Read the model definition and answer for the solid it produces. Units are mm, in the model's axes. A direction names the side the tool comes from. Give positions to 0.01 mm unless a question says otherwise; leave off trailing zeros. Order: outer loops, then holes, each group sorted by start corner. A loop starts at its lowest first (then second) coordinate and runs counter-clockwise, first axis right, second up. Notation, with made-up numbers: M -40,83 L -24,83 A25 cw -24,117 Z; hole C -10,86 d7. An arc over 180 degrees is marked long. Write item = value, one per line. Start each with the question number.
from build123d import *

# Parameters (mm, degrees)
F0_R          = 55
F1_DEPTH      = 250
F1_DEPTH_BACK = 250
F3_DEPTH      = 12
F4_R          = 8
F5_R          = 2


with BuildPart() as f1:
    # F0 (on Right) → F1 (new body, two sides)
    with BuildSketch(Plane.YZ) as f1_sk:
        with Locations((-60, 100)):
            Circle(F0_R)
    extrude(amount=F1_DEPTH)
    extrude(f1_sk.sketch, amount=-F1_DEPTH_BACK)

    # F2 (on Right) → F3 (join)
    with BuildSketch(Plane.YZ):
        with BuildLine():
            ThreePointArc((-29.205577, 167.747019), (-18.607638, 166.4936), (-12.913269, 175.519204))
            Line((-12.913269, 175.519204), (-12.913269, 200))
            Line((-12.913269, 200), (-162.913269, 200))
            Line((-162.913269, 200), (-162.913269, 165))
            Line((-162.913269, 165), (-154.913269, 165))
            Line((-154.913269, 165), (-154.913269, 175))
            Line((-154.913269, 175), (-138.813269, 175))
            Line((-138.813269, 175), (-138.813269, 0))
            Line((-138.813269, 0), (-154.913269, 0))
            Line((-154.913269, 0), (-154.913269, 10))
            Line((-154.913269, 10), (-162.913269, 10))
            Line((-162.913269, 10), (-162.913269, -25))
            Line((-162.913269, -25), (-418.963285, -70.148526))
            Line((-418.963285, -70.148526), (-418.963285, -50.148526))
            ThreePointArc((-418.963285, -50.148526), (-420.690017, -46.368881), (-424.677571, -45.19981))
            ThreePointArc((-424.677571, -45.19981), (-458.697665, -89.391609), (-415.477055, -124.63733))
            Line((-415.477055, -124.63733), (-12.941712, -89.420051))
            ThreePointArc((-12.941712, -89.420051), (-6.440496, -86.214006), (-3.813269, -79.458104))
            Line((-3.813269, -79.458104), (-3.813269, 40.519204))
            ThreePointArc((-3.813269, 40.519204), (-6.742201, 47.590272), (-13.813269, 50.519204))
            Line((-13.813269, 50.519204), (-63.813269, 50.519204))
            ThreePointArc((-63.813269, 50.519204), (-102.704142, 66.628331), (-118.813269, 105.519204))
            Line((-118.813269, 105.519204), (-118.813269, 125))
            ThreePointArc((-118.813269, 125), (-118.518786, 130.683877), (-117.638489, 136.306888))
            Line((-117.638489, 136.306888), (-123.474465, 139.028248))
            Line((-123.474465, 139.028248), (-112.909008, 161.685943))
            Line((-112.909008, 161.685943), (-107.073032, 158.964583))
            ThreePointArc((-107.073032, 158.964583), (-93.364748, 171.38653), (-76.313269, 178.560713))
            Line((-76.313269, 178.560713), (-76.313269, 185))
            Line((-76.313269, 185), (-51.313269, 185))
            Line((-51.313269, 185), (-51.313269, 178.560713))
            ThreePointArc((-51.313269, 178.560713), (-39.646812, 174.406299), (-29.205577, 167.747019))
        make_face()
    extrude(amount=F3_DEPTH)

    # F4
    f4_edges = [f1.edges().sort_by_distance(p)[0] for p in [
        (6, -162.913269, 200),
        (6, -12.913269, 200),
    ]]
    fillet(f4_edges, radius=F4_R)

    # F5
    f5_edges = [f1.edges().sort_by_distance(p)[0] for p in [
        (6, -162.913269, 165),
        (6, -162.913269, 10),
        (6, -154.913269, 165),
        (6, -107.073032, 158.964583),
        (6, -117.638489, 136.306888),
        (6, -76.313269, 178.560713),
        (6, -51.313269, 178.560713),
        (6, -154.913269, 10),
    ]]
    fillet(f5_edges, radius=F5_R)


solid = f1.part
1) Find section A-A on y = -60. Determine the outline of the cut face in (x, z).
2) Find section C-C on x = -151.5. Determine the outline of the cut face in (y, z).
3) For a pull along Z with two mould halves and no side action, classify faces 1 (the face through (6, -147, 175)), 2 (the face through (6, -162.913, -8)), 3 (the face through (6, -87, 200)) as pulls with the +Z half, pulls with the -Z half, needs draft (parallel to the pull), parting line crosses it, or undercut.
4) Find section D-D on z = 59. Determine the outline of the cut face in (x, y).
5) For faces 4 (the face through (5.916, -93.566, 171.258)), 5 (the face through (6, -12.913, 184)), 6 (the face through (5.92, -289.15, -47.26)), determine the directions among +Z, -Z, +X, -X, +Y, -Y from which every point of the face is accessible in a straight line to the end or side of a thin tool.
6) Find section B-B on z = 91.5. Determine the outline of the cut face in (x, y), plus the area to 3 significant figures.
7) Each of these flat-tipped pins is pushed along its axis until it touches: P1, Ø2, axis at x = 8, y = -158, coming from the -Z side; P2, Ø4, axis at x = 8.5, z = 172.5, coming from the +Y side; P3, Ø6, axis at x = 5.5, z = 77.5, coming from the -Y side; P4, Ø3, axis at x = 74, y = -117, coming from the -Z side. Where does it stop, or does it pass through?
8) Find the intervals of material crossed by probe 1 along X at (y, z) = (-347, -63.5); probe 2 along Z at (x, y) = (-165.5, -62); probe 3 along Z at (x, y) = (-190.5, -23), in increasing order. Write a range as [from, to].
Numbers:
q1.outline = M -250,45 L 0,45 L 0,-93.54 L 12,-93.54 L 12,45 L 250,45 L 250,155 L -250,155 Z; M 0,185 L 12,185 L 12,200 L 0,200 Z
q2.outline = C -60,100 d110
q3.face_1 = undercut
q3.face_2 = needs draft
q3.face_3 = pulls with the +Z half
q4.outline = M -250,-96.66 L 0,-96.66 L 0,-138.81 L 12,-138.81 L 12,-96.66 L 250,-96.66 L 250,-23.34 L -250,-23.34 Z
q5.face_4 = +X, -X
q5.face_5 = +Z, +X, -X, +Y
q5.face_6 = +Z, +X, -X
q6.outline = M -250,-114.34 L 250,-114.34 L 250,-5.66 L -250,-5.66 Z; M 0,-138.81 L 12,-138.81 L 12,-117 L 0,-117 Z
q6.area = 54,600 mm2
q7.P1 = -102.2
q7.P2 = -12.97
q7.P3 = -138.81
q7.P4 = through
q8.probe_1 = [0, 12]
q8.probe_2 = [45.04, 154.96]
q8.probe_3 = [59.31, 140.69]
